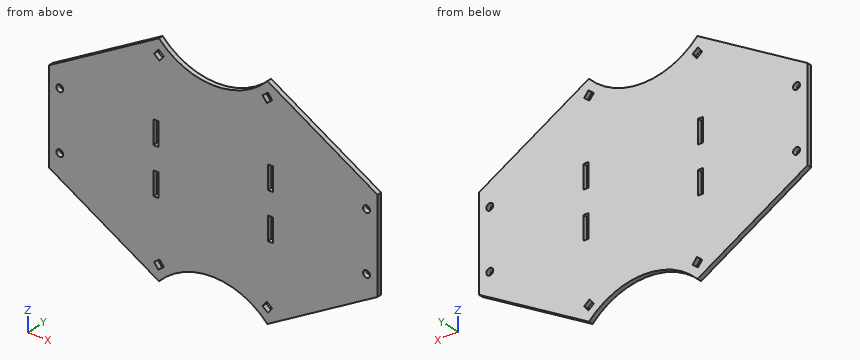
from build123d import *

# Parameters (mm, degrees)
ESQUISSE1_R             = 197.5
BOSS_EXTRU_1_DEPTH      = 4
ENL_V_START             = -1
ESQUISSE3_R             = 3
ENL_V_MAT_EXTRU_2_DEPTH = 6
ENL_V_MAT_EXTRU_5_DEPTH = 5
ESQUISSE6_W             = 4.2
ESQUISSE6_H             = 20.2
ENL_V_MAT_EXTRU_8_DEPTH = 5
ENL_V_MAT_EXTRU_6_DEPTH = 5
CUT_EXTRUDE1_DEPTH      = 5
MIRROR5_COPY_1_DEPTH    = 5
CUT_EXTRUDE2_DEPTH      = 5
MIRROR7_COPY_1_DEPTH    = 5


with BuildPart() as part:
    # Esquisse1 → Boss.-Extru.1 (new body)
    with BuildSketch(Plane(origin=(0, 0, 0), x_dir=(1, 0, 0), z_dir=(0, 1, 0))):
        Circle(ESQUISSE1_R)
    extrude(amount=BOSS_EXTRU_1_DEPTH)

    # Esquisse3 → Enlèv. mat.-Extru.2 (cut)
    with BuildSketch(Plane(origin=(0, 0, 0), x_dir=(1, 0, 0), z_dir=(0, 1, 0)).offset(ENL_V_START)):
        with Locations((-132.97, 25.4)):
            Circle(ESQUISSE3_R)
        with Locations((-132.97, -25.4)):
            Circle(ESQUISSE3_R)
        with BuildLine():
            Line((-180.572007797, 80), (-157.5, 80))
            ThreePointArc((-157.5, 80), (-146.893398282, 75.606601718), (-142.5, 65))
            Line((-142.5, 65), (-142.5, -65))
            ThreePointArc((-142.5, -65), (-146.893398282, -75.606601718), (-157.5, -80))
            Line((-157.5, -80), (-180.572007797, -80))
            ThreePointArc((-180.572007797, -80), (-197.5, 0), (-180.572007797, 80))
        make_face()
    enl_v_mat_extru_2 = extrude(amount=ENL_V_MAT_EXTRU_2_DEPTH, mode=Mode.SUBTRACT)

    # Esquisse4 → Enlèv. mat.-Extru.5 (cut, through all)
    with BuildSketch(Plane(origin=(0, 0, 0), x_dir=(1, 0, 0), z_dir=(0, 1, 0))):
        with BuildLine():
            Line((-107.5, 110), (-107.5, 90))
            ThreePointArc((-107.5, 90), (-104.571067812, 82.928932188), (-97.5, 80))
            Line((-97.5, 80), (-82.5, 80))
            ThreePointArc((-82.5, 80), (-75.428932188, 82.928932188), (-72.5, 90))
            Line((-72.5, 90), (-72.5, 110))
            ThreePointArc((-72.5, 110), (-75.428932188, 117.071067812), (-82.5, 120))
            Line((-82.5, 120), (-97.5, 120))
            ThreePointArc((-97.5, 120), (-104.571067812, 117.071067812), (-107.5, 110))
        make_face()
    enl_v_mat_extru_5 = extrude(amount=ENL_V_MAT_EXTRU_5_DEPTH, mode=Mode.SUBTRACT)

    # Esquisse6 → Enlèv. mat.-Extru.8 (cut, through all)
    with BuildSketch(Plane(origin=(0, 0, 0), x_dir=(1, 0, 0), z_dir=(0, 1, 0))):
        with Locations((-49.6, 20)):
            Rectangle(ESQUISSE6_W, ESQUISSE6_H)
        with Locations((-49.6, -20)):
            Rectangle(ESQUISSE6_W, ESQUISSE6_H)
    enl_v_mat_extru_8 = extrude(amount=ENL_V_MAT_EXTRU_8_DEPTH, mode=Mode.SUBTRACT)

    # Mirror1: Enlèv. mat.-Extru.2, Enlèv. mat.-Extru.5, Enlèv. mat.-Extru.8 across plane
    add(enl_v_mat_extru_2.mirror(Plane(origin=(0, 0, 0), x_dir=(0, 0, 1), z_dir=(1, 0, 0))), mode=Mode.SUBTRACT)
    add(enl_v_mat_extru_5.mirror(Plane(origin=(0, 0, 0), x_dir=(0, 0, 1), z_dir=(1, 0, 0))), mode=Mode.SUBTRACT)
    add(enl_v_mat_extru_8.mirror(Plane(origin=(0, 0, 0), x_dir=(0, 0, 1), z_dir=(1, 0, 0))), mode=Mode.SUBTRACT)

    # Esquisse5 → Enlèv. mat.-Extru.6 (cut, through all)
    with BuildSketch(Plane(origin=(0, 0, 0), x_dir=(1, 0, 0), z_dir=(0, 1, 0))):
        with BuildLine():
            Line((-65, 140), (-65, 186.497319016))
            ThreePointArc((-65, 186.497319016), (0, 197.5), (65, 186.497319016))
            Line((65, 186.497319016), (65, 140))
            ThreePointArc((65, 140), (0, 75), (-65, 140))
        make_face()
    enl_v_mat_extru_6 = extrude(amount=ENL_V_MAT_EXTRU_6_DEPTH, mode=Mode.SUBTRACT)

    # Mirror2: Enlèv. mat.-Extru.6 across plane
    add(enl_v_mat_extru_6.mirror(Plane.XY), mode=Mode.SUBTRACT)

    # Sketch1 → Cut-Extrude1 (cut, through all)
    with BuildSketch(Plane(origin=(0, 4, 0), x_dir=(1, 0, 0), z_dir=(0, 1, 0))):
        Polygon((-47.442047988, -86.219548978), (-51.219548978, -81.557952012), (-46.557952012, -77.780451022), (-42.780451022, -82.442047988), align=None)
    cut_extrude1 = extrude(amount=-CUT_EXTRUDE1_DEPTH, mode=Mode.SUBTRACT)

    # Mirror4: Cut-Extrude1 across plane
    add(cut_extrude1.mirror(Plane.XY), mode=Mode.SUBTRACT)

    # Mirror5: Cut-Extrude1 across plane
    add(cut_extrude1.mirror(Plane(origin=(0, 0, 0), x_dir=(0, 0, 1), z_dir=(1, 0, 0))), mode=Mode.SUBTRACT)

    # Mirror5 copy 1 sketch → Mirror5 copy 1 (cut, through all)
    with BuildSketch(Plane(origin=(0, 4, 0), x_dir=(-1, 0, 0), z_dir=(0, 1, 0))):
        Polygon((-47.442047988, -86.219548978), (-51.219548978, -81.557952012), (-46.557952012, -77.780451022), (-42.780451022, -82.442047988), align=None)
    extrude(amount=-MIRROR5_COPY_1_DEPTH, mode=Mode.SUBTRACT)

    # Sketch3 → Cut-Extrude2 (cut, through all)
    with BuildSketch(Plane(origin=(0, 4, 0), x_dir=(1, 0, 0), z_dir=(0, 1, 0))):
        Polygon((-47.022675211, 95.123859168), (-142.5, 40), (-180.572007797, 80), (-180.572007797, 186.497319016), (-65, 186.497319016), align=None)
    cut_extrude2 = extrude(amount=-CUT_EXTRUDE2_DEPTH, mode=Mode.SUBTRACT)

    # Mirror6: Cut-Extrude2 across plane
    add(cut_extrude2.mirror(Plane.XY), mode=Mode.SUBTRACT)

    # Mirror7: Cut-Extrude2 across plane
    add(cut_extrude2.mirror(Plane(origin=(0, 0, 0), x_dir=(0, 0, 1), z_dir=(1, 0, 0))), mode=Mode.SUBTRACT)

    # Mirror7 copy 1 sketch → Mirror7 copy 1 (cut, through all)
    with BuildSketch(Plane(origin=(0, 4, 0), x_dir=(-1, 0, 0), z_dir=(0, 1, 0))):
        Polygon((-47.022675211, 95.123859168), (-142.5, 40), (-180.572007797, 80), (-180.572007797, 186.497319016), (-65, 186.497319016), align=None)
    extrude(amount=-MIRROR7_COPY_1_DEPTH, mode=Mode.SUBTRACT)


solid = part.part
Work out the finished part from the listing and answer in its coordinate system (mm). Round coordinates to 2 decimals unless told otherwise and drop trailing zeros. Loops run counter-clockwise (first coordinate to the right, second up) from the corner with the lowest first, then second, coordinate; pieces in that order, holes last. Notation, with made-up numbers: M 73.5,-16 L 124.5,-16 A29 ccw 124.5,20 Z; hole C -39.5,48 d8. An arc over 180 degrees is marked long. One line per question, with ' | ' between items. Start each with the question number.
(1) A cutting plane is placed at D-D on x = -92.5. Write down the section's boundary in (y, z).
(2) Find the intervals of material crossed by line 1 (Z direction, x = 132.97, y = 0.9); line 2 (X direction, y = 3.2, z = 43.5); line 3 (Z direction, x = -107, y = 1.75), in increasing order.
(3) Flat-ended cylindrical pins translate along their axes: pin 1 Ø2 at (x, y) = (-48.5, 3) entering from -Z; pin 2 Ø1.5 at (y, z) = (1, -70) entering from -X; pin 3 Ø2 at (x, y) = (-50, 2) entering from +Z. Find the tip coordinate at first contact, or state that the pin passes through.
(4) A cutting plane is placed at B-B on x = 132.97. Write down the section's boundary in (y, z), plus the area to 3 significant figures.
(5) A cutting plane is placed at A-A on z = 25.4. Write down the section's boundary in (x, y).
(6) A cutting plane is placed at C-C on y = 1.4. Give the number of separate pieces and of enclosed holes in the cut face, plus the area to 3 significant figures.
Geometry check:
1) outline: M 0,-68.87 L 4,-68.87 L 4,68.87 L 0,68.87 Z
2) line 1: z = -45.5 to -28.4, -22.4 to 22.4, 28.4 to 45.5 | line 2: x = -136.44 to 136.44 | line 3: z = -60.5 to 60.5
3) pin 1: stops at z = -94.85 | pin 2: stops at x = -91.84 | pin 3: stops at z = 93.98
4) outline: M 0,-45.5 L 4,-45.5 L 4,-28.4 L 0,-28.4 Z; M 0,-22.4 L 4,-22.4 L 4,22.4 L 0,22.4 Z; M 0,28.4 L 4,28.4 L 4,45.5 L 0,45.5 Z | area: 316 mm²
5) outline: M -142.5,0 L -135.97,0 L -135.97,4 L -142.5,4 Z; M -129.97,0 L -51.7,0 L -51.7,4 L -129.97,4 Z; M -47.5,0 L 47.5,0 L 47.5,4 L -47.5,4 Z; M 51.7,0 L 129.97,0 L 129.97,4 L 51.7,4 Z; M 135.97,0 L 142.5,0 L 142.5,4 L 135.97,4 Z
6) separate pieces: 1 | enclosed holes: 12 | area: 40,500 mm²
